The listing builds one solid part. Answer for the finished solid, in the listing's coordinates (mm). Face numbers are marked on the shaded views. A direction names the side the tool comes from. Give positions to 0.01 mm unless a question says otherwise; leave off trailing zeros. Loops run counter-clockwise (first coordinate to the right, second up) from the corner with the lowest first, then second, coordinate; pieces in that order, holes last.
Item 1: Section A-A, the plane x = 0 is taken. Give the vertices of the cut face in (y, z), and give its area (3 significant figures).
Item 2: Each of these flat-tipped pins is pushed along its axis until it touches: pin 1 Ø6 at (x, z) = (-5, -0.5) entering from +Y; pin 2 Ø6 at (x, y) = (-7, -7.5) entering from +Z; pin 3 Ø10 at (y, z) = (-7, 4) entering from +X. Where does it stop, or does it pass through?
Item 3: Consider line 1 along Y through (x, z) = (0, 12.6); line 2 along Z through (x, y) = (-5.5, 5.25); line 3 along Z through (x, y) = (4.5, 9). Determine where each line is inside the solid, lowest interval first.
Item 4: Section D-D, the plane y = -5 is taken. Give the vertices of the cut face in (x, z), and give its area (3 significant figures).
Item 5: A tool of negligible diameter and unlimited length cuts with its end or side. For the marked faces 1 and 2, from which of +Z, -Z, +X, -X, +Y, -Y can it reach the whole face along a straight path? Write none if from no direction.
Item 6: Section C-C, the plane z = 10.75 is taken. Give the vertices of the cut face in (x, y), and give its area (3 significant figures).
Item 7: The mould has two halves that part along X. Classify the marked faces 3, 4 and 5: pulls with the +X half, pulls with the -X half, needs draft (parallel to the pull), parting line crosses it, or undercut.
from build123d import *

# Parameters (mm, degrees)
CROQUIS1_R              = 11
SALIENTE_EXTRUIR1_DEPTH = 12.8
CROQUIS2_R              = 8.8
CROQUIS2_R_2            = 6
CORTAR_EXTRUIR1_DEPTH   = 0.4
CROQUIS3_R              = 4
SALIENTE_EXTRUIR2_DEPTH = 5.6


with BuildPart() as part:
    # Croquis1 → Saliente-Extruir1 (new body)
    with BuildSketch(Plane.XY):
        Circle(CROQUIS1_R)
    extrude(amount=SALIENTE_EXTRUIR1_DEPTH)

    # Croquis2 → Cortar-Extruir1 (cut)
    with BuildSketch(Plane.XY.offset(12.8)):
        Circle(CROQUIS2_R)
        Circle(CROQUIS2_R_2, mode=Mode.SUBTRACT)
    cortar_extruir1 = extrude(amount=-CORTAR_EXTRUIR1_DEPTH, mode=Mode.SUBTRACT)

    # Croquis3 → Saliente-Extruir2 (add)
    with BuildSketch(Plane.XY.offset(12.8)):
        Circle(CROQUIS3_R)
    saliente_extruir2 = extrude(amount=SALIENTE_EXTRUIR2_DEPTH)

    # Simetría1: Cortar-Extruir1, Saliente-Extruir2 across plane
    add(cortar_extruir1.mirror(Plane.XY.offset(6.4)), mode=Mode.SUBTRACT)
    add(saliente_extruir2.mirror(Plane.XY.offset(6.4)))


solid = part.part
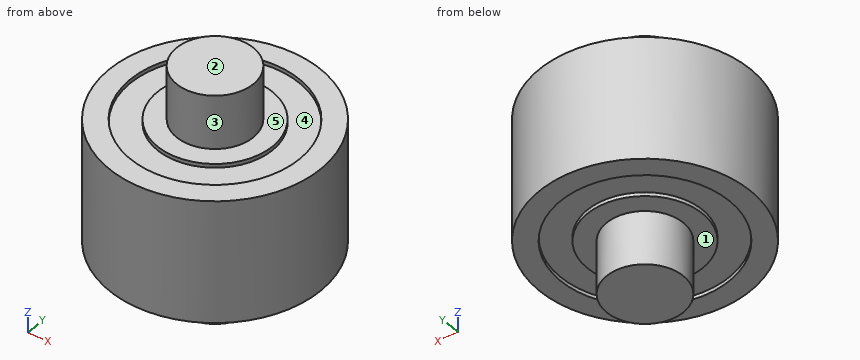
Worked answers:
1. outline: (-11, 0) - (-8.8, 0) - (-8.8, 0.4) - (-6, 0.4) - (-6, 0) - (-4, 0) - (-4, -5.6) - (4, -5.6) - (4, 0) - (6, 0) - (6, 0.4) - (8.8, 0.4) - (8.8, 0) - (11, 0) - (11, 12.8) - (8.8, 12.8) - (8.8, 12.4) - (6, 12.4) - (6, 12.8) - (4, 12.8) - (4, 18.4) - (-4, 18.4) - (-4, 12.8) - (-6, 12.8) - (-6, 12.4) - (-8.8, 12.4) - (-8.8, 12.8) - (-11, 12.8) - close
1. area: 367 mm2
2. pin 1: stops at y = 10.81
2. pin 2: stops at z = 12.8
2. pin 3: stops at x = 10.82
3. line 1: y = -11 to -8.8, -6 to 6, 8.8 to 11
3. line 2: z = 0.4 to 12.4
3. line 3: z = 0 to 12.8
4. outline: (-9.8, 0) - (-7.24, 0) - (-7.24, 0.4) - (-3.32, 0.4) - (-3.32, 0) - (3.32, 0) - (3.32, 0.4) - (7.24, 0.4) - (7.24, 0) - (9.8, 0) - (9.8, 12.8) - (7.24, 12.8) - (7.24, 12.4) - (3.32, 12.4) - (3.32, 12.8) - (-3.32, 12.8) - (-3.32, 12.4) - (-7.24, 12.4) - (-7.24, 12.8) - (-9.8, 12.8) - close
4. area: 245 mm2
5. face 1: -Z
5. face 2: +Z, +X, -X, +Y, -Y
6. outline: circle Ø22 at (0, 0)
6. area: 380 mm2
7. face 3: parting line crosses it
7. face 4: undercut
7. face 5: needs draft
